Drawing for the job (mm, zero at the part's lowest x, y, z). A direction names the side the tool comes from. Give positions to 0.01 mm unless a question says otherwise; leave off trailing zeros. Loops run counter-clockwise (first coordinate to the right, second up) from the corner with the lowest first, then second, coordinate; pieces in that order, holes last. Notation, with made-up numbers: (41, -14.5) -> (69, -14.5) arc R28 cw to (69, 24.5) -> close; hole circle Ø2 at (67, 8.25). An arc over 180 degrees is marked (long way). Answer in a Markdown table with one row per item. Add a question column.
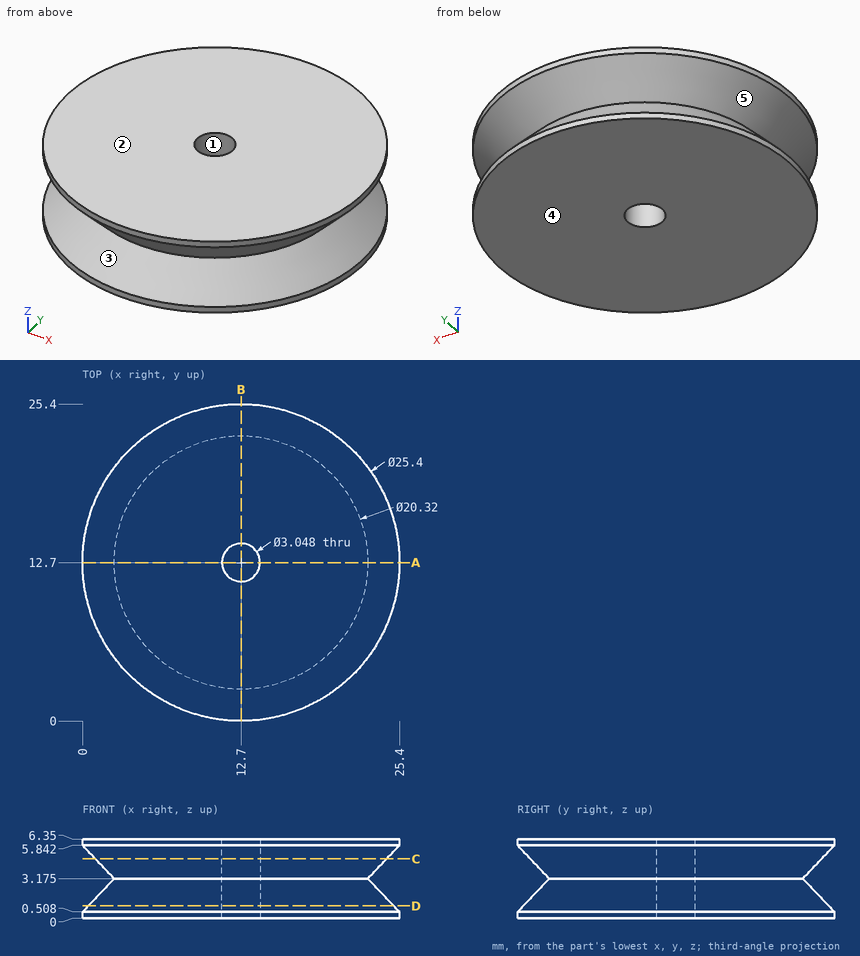
(1) Saw through at A-A, the plane y = 12.7. List the corners of the cut face in (x, z) (3 decimals), then the cut area to 3 significant figures.
(2) Saw through at D-D, the plane z = 1. List the corners of the cut face in (x, y).
(3) 3-axis set-ups, long thin cutter, end or side, ignore diameter. For the marked faces 4 and 5: which of +Z, -Z, +X, -X, +Y, -Y reach the whole face in a straight line?
(4) Wall check: line 1 along Z through (x, y) = (3.25, 5.25); line 2 along Y through (x, z) = (12.7, 3); line 3 along Z through (x, y) = (23, 18.5). Give the ranges that are in metal, low to high. Write a range as from..to.
(5) Two-plate mould, pull along X, no slides. Class the marked faces 1, 2 and 3: released by +X, released by -X, zero draft, split by the parting line, or undercut.
(6) Saw through at C-C, the plane z = 4.75. List the corners of the cut face in (x, y).
(7) Flat gauge pin, fed straight in: pin 1 Ø2 at (x, z) = (10.5, 4) entering from +Y. Where does the tip first touch, or does it go through?
Worked answers:
| question | item | result |
|---|---|---|
| 1 | outline | (0, 0) -> (11.176, 0) -> (11.176, 6.35) -> (0, 6.35) -> (0, 5.842) -> (2.54, 3.175) -> (0, 0.508) -> close; (14.224, 0) -> (25.4, 0) -> (25.4, 0.508) -> (22.86, 3.175) -> (25.4, 5.842) -> (25.4, 6.35) -> (14.224, 6.35) -> close |
| 1 | area | 128 mm^2 |
| 2 | outline | circle Ø24.46 at (12.7, 12.7); hole circle Ø3.05 at (12.7, 12.7) |
| 3 | face 4 | -Z, +X, -X, +Y, -Y |
| 3 | face 5 | none |
| 4 | line 1 | 0..1.21, 5.14..6.35 |
| 4 | line 2 | 2.37..11.18, 14.22..23.03 |
| 4 | line 3 | 0..1.43, 4.92..6.35 |
| 5 | face 1 | undercut |
| 5 | face 2 | zero draft |
| 5 | face 3 | split by the parting line |
| 6 | outline | circle Ø23.32 at (12.7, 12.7); hole circle Ø3.05 at (12.7, 12.7) |
| 7 | pin 1 | y = 24.41 |
